Input: part model. Units: mm. Frame: model coordinates. Give positions to 0.01 mm unless a question says otherwise; leave off trailing zeros. Loops run counter-clockwise (first coordinate to the right, second up) from the corner with the lowest first, then second, coordinate; pieces in that order, holes last. Notation, with made-up numbers: M 77.5,-6 L 98.5,-6 A14 cw 98.5,17 Z; hole C -40,70 d10. An arc over 180 degrees is marked long. Use CSV: the item, a comma, the result in double quotes. Start each with the question number.
Q1. Pull-direction query (Y, two-part tool) for faces 1 (the flat face through (3, -1, 1)), 2 (the flat face through (-2.647, 1.785, 0.507)); classes: released by +Y, released by -Y, zero draft, split by the parting line, or undercut.
Q2. Material intervals for line 1 along Y through (x, z) = (-2.75, 0.2); line 2 along X through (y, z) = (-3, 0.2); line 3 along X through (y, z) = (2, 0.85), sorted ascending.
Q3. Section D-D, the plane x = 2.75. Output: boundary loops of the cut face in (y, z), plus the area to 3 significant figures.
Q4. Section A-A, the plane x = 0. Output: boundary loops of the cut face in (y, z).
from build123d import *

# Parameters (mm, degrees)
CYLINDER003_R          = 2
CYLINDER003_DEPTH      = 10
CYLINDER002_W          = 3.75
CYLINDER002_H          = 10
CYLINDER002_ANGLE      = 22.5
CUT001_PLACEMENT_ANGLE = -11.5
ARRAY_COUNT            = 8
CYLINDER001_R          = 2.65
CYLINDER001_DEPTH      = 2
CYLINDER_R             = 5
CYLINDER_DEPTH         = 1


with BuildPart() as vaciado_sector:
    # Cylinder003 → Cylinder003 (new body)
    with BuildSketch(Plane.XY):
        Circle(CYLINDER003_R)
    extrude(amount=CYLINDER003_DEPTH)


with BuildPart() as obj1:
    # Cylinder002 → Cylinder002 (revolve)
    with BuildSketch(Plane.XZ):
        with Locations((1.875, 5)):
            Rectangle(CYLINDER002_W, CYLINDER002_H)
    revolve(axis=Axis((0, 0, 0), (0, 0, 1)), revolution_arc=CYLINDER002_ANGLE)

    # Cut001: cut vaciado sector
    add(vaciado_sector.part, mode=Mode.SUBTRACT)


with BuildPart() as obj1_1:
    # Cut001 placement: moved
    add(obj1.part.moved(Location((0, 0, -5))).rotate(Axis((0, 0, -5), (0, 0, 1)), CUT001_PLACEMENT_ANGLE))

    # Array: obj1 ×8 about axis
    array_axis = Axis((0, 0, 0), (0, 0, 1))


with BuildPart() as obj1_2:
    add(obj1_1.part)
    for i in range(1, ARRAY_COUNT):
        add(obj1_1.part.rotate(array_axis, i * 360 / ARRAY_COUNT))


with BuildPart() as obj2:
    # Cylinder001 → Cylinder001 (new body)
    with BuildSketch(Plane.XY.offset(-0.5)):
        Circle(CYLINDER001_R)
    extrude(amount=CYLINDER001_DEPTH)


with BuildPart() as obj3:
    # Cylinder → Cylinder (new body)
    with BuildSketch(Plane.XY):
        Circle(CYLINDER_R)
    extrude(amount=CYLINDER_DEPTH)

    # Cut: cut obj2
    add(obj2.part, mode=Mode.SUBTRACT)

    # Cut002: cut obj1
    add(obj1_2.part, mode=Mode.SUBTRACT)


solid = obj3.part
A:
1,face 1,"zero draft"
1,face 2,"undercut"
2,line 1,"-4.18 to -2.55, -1.82 to -0.53, 0.56 to 1.85, 2.55 to 4.18"
2,line 2,"-4 to -2.25, -2.02 to -0.61, 0.58 to 1.99, 2.25 to 4"
2,line 3,"-4.58 to -2.97, 3.02 to 4.58"
3,outline,"M -4.18,0 L -2.55,0 L -2.55,1 L -4.18,1 Z; M -1.85,0 L -0.56,0 L -0.56,1 L -1.85,1 Z; M 0.53,0 L 1.82,0 L 1.82,1 L 0.53,1 Z; M 2.55,0 L 4.18,0 L 4.18,1 L 2.55,1 Z"
3,area,"5.83 mm^2"
4,outline,"M -5,0 L -3.75,0 L -3.75,1 L -5,1 Z; M 3.75,0 L 5,0 L 5,1 L 3.75,1 Z"
